Part print with two shaded views. Sizes in mm from the minimum x, y, z corner. A direction names the side the tool comes from. Round coordinates to 2 decimals unless told otherwise and drop trailing zeros. Order: outer loops, then holes, each group sorted by start corner. A loop starts at its lowest first (then second) coordinate and runs counter-clockwise, first axis right, second up. Notation, with made-up numbers: (-22, -28) - (-10, -28) arc R30 ccw to (-10, -1) - close; hole circle Ø8 at (77, 12). An arc over 180 degrees is marked (long way). Use one line per item in the form item = value.
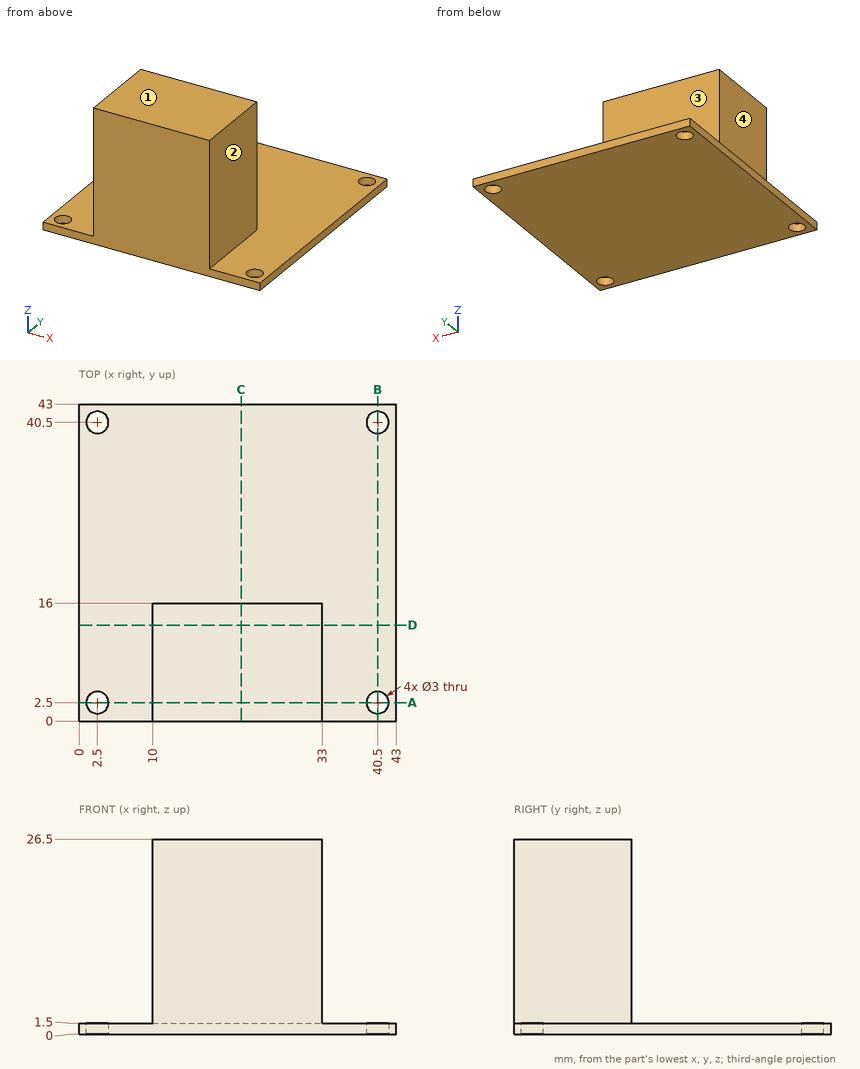
(1) Probe probe 1 along Y at (x, z) = (40.5, 0.8); probe 2 along Y at (x, z) = (16, 22); probe 3 along Z at (x, y) = (4.5, 16). List the from-to ranges inside material, lowest first. Write a range as [from, to].
Report:
probe_1 = [0, 1], [4, 39], [42, 43]
probe_2 = [0, 16]
probe_3 = [0, 1.5]
(2) Slice it at D-D on y = 13. Give the cut face in (x, z), then the cut area to 4 significant figures.
Report:
outline = (0, 0) - (43, 0) - (43, 1.5) - (33, 1.5) - (33, 26.5) - (10, 26.5) - (10, 1.5) - (0, 1.5) - close
area = 639.5 mm2
(3) Tool access for the marked faces 1, 2, 3 and 4: list every direction of +Z, -Z, +X, -X, +Y, -Y with a clear straight run to the whole face (end or side of a thin tool).
Report:
face_1 = +Z, +X, -X, +Y, -Y
face_2 = +Z, +X, +Y, -Y
face_3 = +Z, +X, -X, +Y
face_4 = +Z, -X, +Y, -Y
(4) Pin check, flat tips, straight feed: pin 1 (2.5 mm diameter, centred on x = 2.5, y = 2.5, fed in from -Z); pin 2 (5 mm diameter, centred on y = 6, z = 18, fed in from -X); pin 3 (6 mm diameter, centred on x = 31, y = 33.5, fed in from +Z); pin 4 (11.5 mm diameter, centred on x = 21.5, z = 13, fed in from +Y). Stop position of each tip, or through.
Report:
pin_1 = through
pin_2 = 10
pin_3 = 1.5
pin_4 = 16
(5) Slice it at A-A on y = 2.5. Give the cut face in (x, z).
Report:
outline = (0, 0) - (1, 0) - (1, 1.5) - (0, 1.5) - close; (4, 0) - (39, 0) - (39, 1.5) - (33, 1.5) - (33, 26.5) - (10, 26.5) - (10, 1.5) - (4, 1.5) - close; (42, 0) - (43, 0) - (43, 1.5) - (42, 1.5) - close
(6) Slice it at C-C on x = 22. Give the cut face in (y, z).
Report:
outline = (0, 0) - (43, 0) - (43, 1.5) - (16, 1.5) - (16, 26.5) - (0, 26.5) - close
(7) Slice it at B-B on x = 40.5. Give the cut face in (y, z), then the cut area to 3 significant figures.
Report:
outline = (0, 0) - (1, 0) - (1, 1.5) - (0, 1.5) - close; (4, 0) - (39, 0) - (39, 1.5) - (4, 1.5) - close; (42, 0) - (43, 0) - (43, 1.5) - (42, 1.5) - close
area = 55.5 mm2
